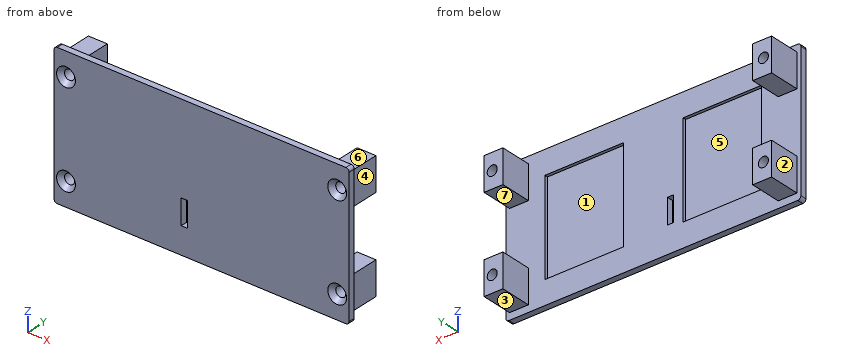
from build123d import *

# Parameters (mm, degrees)
SKETCH1_W                                           = 94
SKETCH1_H                                           = 45
BOSS_EXTRUDE1_DEPTH                                 = 2
FILLET1_R                                           = 1
SKETCH2_W                                           = 6
SKETCH2_H                                           = 10.6
BOSS_EXTRUDE2_DEPTH                                 = 10
SKETCH8_W                                           = 25
SKETCH8_H                                           = 30
CUT_EXTRUDE1_DEPTH                                  = 1
CSK_FOR_M5_COUNTERSUNK_FLAT_HEAD_SCREW1_D           = 3.2
CSK_FOR_M5_COUNTERSUNK_FLAT_HEAD_SCREW1_DEPTH       = 15
CSK_FOR_M5_COUNTERSUNK_FLAT_HEAD_SCREW1_CSINK_D     = 6
CSK_FOR_M5_COUNTERSUNK_FLAT_HEAD_SCREW1_CSINK_ANGLE = 90
CUT_EXTRUDE2_REACH                                  = 55.472
SKETCH9_W                                           = 2
SKETCH9_H                                           = 8


with BuildPart() as part:
    # Sketch1 → Boss-Extrude1 (new body)
    with BuildSketch(Plane(origin=(0, 0, 0), x_dir=(1, 0, 0), z_dir=(0, 1, 0))):
        Rectangle(SKETCH1_W, SKETCH1_H)
    extrude(amount=BOSS_EXTRUDE1_DEPTH)

    # Fillet1
    fillet1_edges = [part.edges().sort_by_distance(p)[0] for p in [
        (-47, 1, 22.5),
        (47, 1, 22.5),
        (47, 1, -22.5),
        (-47, 1, -22.5),
    ]]
    fillet(fillet1_edges, radius=FILLET1_R)

    # Sketch2 → Boss-Extrude2 (add)
    with BuildSketch(Plane(origin=(0, 2, 0), x_dir=(1, 0, 0), z_dir=(0, 1, 0))):
        with Locations((-42.8, -15)):
            Rectangle(SKETCH2_W, SKETCH2_H)
        with Locations((-42.8, 15)):
            Rectangle(SKETCH2_W, SKETCH2_H)
    boss_extrude2 = extrude(amount=BOSS_EXTRUDE2_DEPTH)

    # Sketch8 → Cut-Extrude1 (cut)
    with BuildSketch(Plane(origin=(0, 2, 0), x_dir=(1, 0, 0), z_dir=(0, 1, 0))):
        with Locations((-22, 0)):
            Rectangle(SKETCH8_W, SKETCH8_H)
    cut_extrude1 = extrude(amount=-CUT_EXTRUDE1_DEPTH, mode=Mode.SUBTRACT)

    # CSK for M5 Countersunk Flat Head Screw1
    with Locations(Plane(origin=(-43.2, 0, -15), x_dir=(0, 0, -1), z_dir=(0, -1, 0))):
        with Locations((0, 0), (-30, 0)):
            csk_for_m5_countersunk_flat_head_screw1 = CounterSinkHole(CSK_FOR_M5_COUNTERSUNK_FLAT_HEAD_SCREW1_D / 2, CSK_FOR_M5_COUNTERSUNK_FLAT_HEAD_SCREW1_CSINK_D / 2, depth=CSK_FOR_M5_COUNTERSUNK_FLAT_HEAD_SCREW1_DEPTH, counter_sink_angle=CSK_FOR_M5_COUNTERSUNK_FLAT_HEAD_SCREW1_CSINK_ANGLE)

    # Mirror1: Boss-Extrude2, Cut-Extrude1, CSK for M5 Countersunk Flat Head Screw1 across plane
    add(boss_extrude2.mirror(Plane.ZY))
    add(cut_extrude1.mirror(Plane.ZY), mode=Mode.SUBTRACT)
    add(csk_for_m5_countersunk_flat_head_screw1.mirror(Plane.ZY), mode=Mode.SUBTRACT)

    # Sketch9 → Cut-Extrude2 (cut, up to next)
    with BuildSketch(Plane.XZ, mode=Mode.PRIVATE) as cut_extrude2_sk1:
        with Locations((-5.5, -10)):
            Rectangle(SKETCH9_W, SKETCH9_H)
    cut_extrude2_tool1 = extrude(cut_extrude2_sk1.sketch, amount=-CUT_EXTRUDE2_REACH, mode=Mode.PRIVATE) & part.part
    add(cut_extrude2_tool1.solids().sort_by_distance((-5.5, 0, -10))[0], mode=Mode.SUBTRACT)


solid = part.part
Input: part model. Units: mm. Frame: model coordinates. Face numbers are marked on the shaded views. A direction names the side the tool comes from. Round coordinates to 2 decimals unless told otherwise and drop trailing zeros. Order: outer loops, then holes, each group sorted by start corner. A loop starts at its lowest first (then second) coordinate and runs counter-clockwise, first axis right, second up.
1. Material intervals for line 1 (X direction, y = 6.5, z = -15); line 2 (Z direction, x = -43.2, y = 7.75); line 3 (X direction, y = 9, z = 15.5), sorted ascending.
The answers:
line 1: x = -45.8 to -44.8, -41.6 to -39.8, 39.8 to 41.6, 44.8 to 45.8
line 2: z = -20.3 to -16.6, -13.4 to -9.7, 9.7 to 13.4, 16.6 to 20.3
line 3: x = -45.8 to -44.72, -41.68 to -39.8, 39.8 to 41.68, 44.72 to 45.8
2. Cut plane C-C, the plane z = 0. Output: boundary loops of the cut face in (x, y), then the cut area to 3 significant figures.
The answers:
outline: (-47, 0) - (47, 0) - (47, 2) - (34.5, 2) - (34.5, 1) - (9.5, 1) - (9.5, 2) - (-9.5, 2) - (-9.5, 1) - (-34.5, 1) - (-34.5, 2) - (-47, 2) - close
area: 138 mm2
3. Cut plane B-B, the plane y = 10.5. Output: boundary loops of the cut face in (x, z).
The answers:
outline: (-45.8, -20.3) - (-39.8, -20.3) - (-39.8, -9.7) - (-45.8, -9.7) - close; (-45.8, 9.7) - (-39.8, 9.7) - (-39.8, 20.3) - (-45.8, 20.3) - close; (39.8, -20.3) - (45.8, -20.3) - (45.8, -9.7) - (39.8, -9.7) - close; (39.8, 9.7) - (45.8, 9.7) - (45.8, 20.3) - (39.8, 20.3) - close; hole circle Ø3.2 at (-43.2, -15); hole circle Ø3.2 at (-43.2, 15); hole circle Ø3.2 at (43.2, -15); hole circle Ø3.2 at (43.2, 15)
4. Set-up query: the marked faces 1, 2 and 3. Return all of +Z, -Z, +X, -X, +Y, -Y with unobstructed straight access to the full face (end or side cutting, diameter ignored); none if empty.
The answers:
face 1: +Y
face 2: +Z, -Z, -X, +Y
face 3: -Z, +X, -X, +Y
5. Cut plane D-D, the plane x = -10.5. Output: boundary loops of the cut face in (y, z).
The answers:
outline: (0, -22.5) - (2, -22.5) - (2, -15) - (1, -15) - (1, 15) - (2, 15) - (2, 22.5) - (0, 22.5) - close
6. Pin query (flat end, axial travel): P1, Ø2, axis at y = 5, z = -15.5, coming from the +X side; P2, Ø3, axis at x = -12, z = -9.5, coming from the +Y side; P3, Ø5, axis at x = -18, z = -11.5, coming from the -Y side; P4, Ø8, axis at x = 34.5, z = -9.5, coming from the +Y side. Return the tip coordinate at first contact, or that it passes through.
The answers:
P1: stops at x = 45.8
P2: stops at y = 1
P3: stops at y = 0
P4: stops at y = 2
7. Mould query, pull axis Z, two halves, no side actions, for the marked faces 4, 5, 6 and 7. Classes: released by +Z, released by -Z, zero draft, split by the parting line, or undercut.
The answers:
face 4: zero draft
face 5: undercut
face 6: released by +Z
face 7: undercut
8. Cut plane A-A, the plane x = 43.2. Output: boundary loops of the cut face in (y, z), then the cut area to 3 significant figures.
The answers:
outline: (0, -22.5) - (2, -22.5) - (2, -20.3) - (12, -20.3) - (12, -16.6) - (1.4, -16.6) - (0, -18) - close; (0, -12) - (1.4, -13.4) - (12, -13.4) - (12, -9.7) - (2, -9.7) - (2, 9.7) - (12, 9.7) - (12, 13.4) - (1.4, 13.4) - (0, 12) - close; (0, 18) - (1.4, 16.6) - (12, 16.6) - (12, 20.3) - (2, 20.3) - (2, 22.5) - (0, 22.5) - close
area: 221 mm2
